Read the model definition and answer for the solid it produces. Units are mm, in the model's axes. Give positions to 0.01 mm unless a question says otherwise; leave off trailing zeros. Loops run counter-clockwise (first coordinate to the right, second up) from the corner with the lowest first, then second, coordinate; pieces in that order, holes last. Notation, with made-up numbers: (30.25, 78) -> (89.25, 78) arc R24 cw to (89.25, 97) -> close; hole circle Ø6 at (-24.5, 0). An arc over 180 degrees is marked (long way). Write each question's results on one line, items separated by ' | '. Start each with the question number.
Item 1: Each of these flat-tipped pins is pushed along its axis until it touches: P1, Ø3, axis at x = -62.76, y = -56.51, coming from the -Z side; P2, Ø0.6, axis at x = 79.5, z = 2, coming from the +Y side; P3, Ø6.5, axis at x = 62.76, y = -56.51, coming from the -Z side; P4, Ø1, axis at x = -24.5, z = 0.5, coming from the +Y side. Where does it stop, or does it pass through?
Item 2: Section A-A on y = 0 is taken. Write down the section's boundary in (x, z) (1 decimal).
Item 3: Find the intervals of material crossed by line 1 (X direction, y = 1.5, z = 0.15); line 2 (Y direction, x = -77, z = 1.4); line 3 (Y direction, x = -57.5, z = 1.1), in increasing order.
Item 4: Section B-B on x = 24.5 is taken. Write down the section's boundary in (y, z) (3 decimals), and give its area (3 significant figures).
Item 5: Section C-C on z = 1.35 is taken. State how many separate pieces and enclosed holes the cut face has, and give its area (3 significant figures).
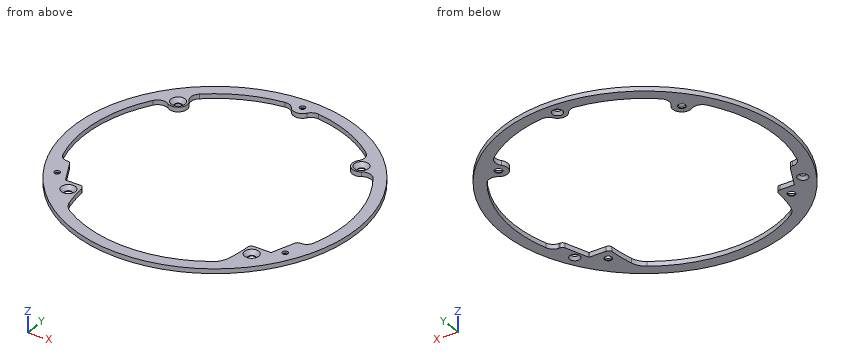
```python
from build123d import *

# Parameters (mm, degrees)
SKETCH1_R                 = 98.1075
SKETCH1_R_2               = 90.17
BOSS_EXTRUDE1_DEPTH       = 3.175
BOSS_EXTRUDE2_START       = -3.175
BOSS_EXTRUDE2_DEPTH       = 3.175
BOSS_EXTRUDE3_START       = -3.175
BOSS_EXTRUDE3_DEPTH       = 3.175
BOSS_EXTRUDE5_DEPTH       = 3.175
MIRROR2_START             = -3.175
MIRROR2_COPY_1_DEPTH      = 3.175
CIRPATTERN1_COUNT         = 3
FILLET1_R                 = 3.175
BOSS_EXTRUDE6_START       = -3.175
BOSS_EXTRUDE6_DEPTH       = 3.175
FILLET2_R                 = 6.35
F_6_CLEARANCE_HOLE1_D     = 3.7973
F_6_CLEARANCE_HOLE1_DEPTH = 6.35
F_6_CLEARANCE_HOLE1_TIP   = 1.140824014
CUT_EXTRUDE1_DEPTH        = 139.781280213
FILLET3_R                 = 2.54


with BuildPart() as part:
    # Sketch1 → Boss-Extrude1 (new body)
    with BuildSketch(Plane.XY):
        Circle(SKETCH1_R)
        Circle(SKETCH1_R_2, mode=Mode.SUBTRACT)
    extrude(amount=BOSS_EXTRUDE1_DEPTH)

    # Sketch2 → Boss-Extrude2 (add)
    with BuildSketch(Plane.XY.offset(3.175).offset(BOSS_EXTRUDE2_START)):
        with BuildLine():
            ThreePointArc((-5.291472464, 86.659612676), (0, 83.82), (5.291472464, 86.659612676))
            ThreePointArc((5.291472464, 86.659612676), (7.940261692, 88.923194985), (11.38468318, 89.448409091))
            ThreePointArc((11.38468318, 89.448409091), (0, 90.17), (-11.38468318, 89.448409091))
            ThreePointArc((-11.38468318, 89.448409091), (-7.940261692, 88.923194985), (-5.291472464, 86.659612676))
        make_face()
    boss_extrude2 = extrude(amount=BOSS_EXTRUDE2_DEPTH)

    # Sketch9 → Boss-Extrude3 (add)
    with BuildSketch(Plane.XY.offset(3.175).offset(BOSS_EXTRUDE3_START)):
        with BuildLine():
            ThreePointArc((66.212341469, -51.332340799), (58.137705987, -52.347425597), (57.972211169, -60.483932635))
            ThreePointArc((57.972211169, -60.483932635), (59.462085873, -65.336411741), (57.068521986, -69.812697257))
            ThreePointArc((57.068521986, -69.812697257), (67.009368913, -60.335506775), (75.395540901, -49.458480691))
            ThreePointArc((75.395540901, -49.458480691), (71.1939725, -52.306831631), (66.212341469, -51.332340799))
        make_face()
    boss_extrude3 = extrude(amount=BOSS_EXTRUDE3_DEPTH)

    # Sketch11 → Boss-Extrude5 (add)
    with BuildSketch(Plane.XY):
        with BuildLine():
            ThreePointArc((-60.552516274, -19.396575562), (-63.5, -44.45), (-60.552516274, -69.503424438))
            ThreePointArc((-60.552516274, -69.503424438), (-57.572960629, -76.08635224), (-52.356101558, -81.086059404))
            ThreePointArc((-52.356101558, -81.086059404), (0, -96.52), (52.356101558, -81.086059404))
            ThreePointArc((52.356101558, -81.086059404), (57.572960629, -76.08635224), (60.552516274, -69.503424438))
            ThreePointArc((60.552516274, -69.503424438), (63.5, -44.45), (60.552516274, -19.396575562))
            ThreePointArc((60.552516274, -19.396575562), (57.572960629, -12.81364776), (52.356101558, -7.813940596))
            ThreePointArc((52.356101558, -7.813940596), (0, 7.62), (-52.356101558, -7.813940596))
            ThreePointArc((-52.356101558, -7.813940596), (-57.572960629, -12.81364776), (-60.552516274, -19.396575562))
        make_face()
        with BuildLine():
            ThreePointArc((48.911621193, -13.148549768), (0, 1.27), (-48.911621193, -13.148549768))
            ThreePointArc((-48.911621193, -13.148549768), (-52.38952724, -16.481687877), (-54.37589767, -20.870306412))
            ThreePointArc((-54.37589767, -20.870306412), (-57.15, -44.45), (-54.37589767, -68.029693588))
            ThreePointArc((-54.37589767, -68.029693588), (-52.38952724, -72.418312123), (-48.911621193, -75.751450232))
            ThreePointArc((-48.911621193, -75.751450232), (0, -90.17), (48.911621193, -75.751450232))
            ThreePointArc((48.911621193, -75.751450232), (52.38952724, -72.418312123), (54.37589767, -68.029693588))
            ThreePointArc((54.37589767, -68.029693588), (57.15, -44.45), (54.37589767, -20.870306412))
            ThreePointArc((54.37589767, -20.870306412), (52.38952724, -16.481687877), (48.911621193, -13.148549768))
        make_face(mode=Mode.SUBTRACT)
    extrude(amount=BOSS_EXTRUDE5_DEPTH)

    # Sketch3 → CSK for #10 Flat Head Machine Screw1 (revolve, cut)
    with BuildSketch(Plane(origin=(62.762296236, -56.51142536, 3.175), x_dir=(0, -1, 0), z_dir=(1, 0, 0))):
        Polygon((0, 0), (0, 3.175), (2.5527, 3.175), (2.5527, 2.688180894), (4.8895, 0), align=None)
    csk_for_10_flat_head_machine_screw1 = revolve(axis=Axis((62.762296236, -56.51142536, 9.525), (0, 0, -1)), mode=Mode.SUBTRACT)

    # Sketch7 → CSK for #6 Flat Head Machine Screw1 (revolve, cut)
    with BuildSketch(Plane(origin=(0, 90.17, 0), x_dir=(0, 1, 0), z_dir=(1, 0, 0))):
        Polygon((0, 0), (0, 3.175), (1.89865, 3.175), (1.89865, 1.891953401), (3.5433, 0), align=None)
    csk_for_6_flat_head_machine_screw1 = revolve(axis=Axis((0, 90.17, -6.35), (0, 0, 1)), mode=Mode.SUBTRACT)

    # Mirror1: Boss-Extrude3, CSK for #10 Flat Head Machine Screw1 across plane
    add(boss_extrude3.mirror(Plane.ZX))
    add(csk_for_10_flat_head_machine_screw1.mirror(Plane.ZX), mode=Mode.SUBTRACT)

    # Mirror2: Boss-Extrude3, CSK for #10 Flat Head Machine Screw1 across plane
    add(boss_extrude3.mirror(Plane(origin=(0, 0, 0), x_dir=(0, 0, 1), z_dir=(1, 0, 0))))
    add(csk_for_10_flat_head_machine_screw1.mirror(Plane(origin=(0, 0, 0), x_dir=(0, 0, 1), z_dir=(1, 0, 0))), mode=Mode.SUBTRACT)

    # Mirror2 copy 1 sketch → Mirror2 copy 1 (add)
    with BuildSketch(Plane(origin=(0, 0, 3.175), x_dir=(-1, 0, 0), z_dir=(0, 0, 1)).offset(MIRROR2_START)):
        with BuildLine():
            ThreePointArc((66.212341469, -51.332340799), (58.137705987, -52.347425597), (57.972211169, -60.483932635))
            ThreePointArc((57.972211169, -60.483932635), (59.462085873, -65.336411741), (57.068521986, -69.812697257))
            ThreePointArc((57.068521986, -69.812697257), (67.009368913, -60.335506775), (75.395540901, -49.458480691))
            ThreePointArc((75.395540901, -49.458480691), (71.1939725, -52.306831631), (66.212341469, -51.332340799))
        make_face()
    extrude(amount=MIRROR2_COPY_1_DEPTH)

    # Mirror2 copy 2 sketch → Mirror2 copy 2 (revolve, cut)
    with BuildSketch(Plane(origin=(-62.762296236, 56.51142536, 3.175), x_dir=(0, 1, 0), z_dir=(-1, 0, 0))):
        Polygon((0, 0), (0, 3.175), (2.5527, 3.175), (2.5527, 2.688180894), (4.8895, 0), align=None)
    revolve(axis=Axis((-62.762296236, 56.51142536, 9.525), (0, 0, -1)), mode=Mode.SUBTRACT)

    # CirPattern1: Boss-Extrude2, CSK for #6 Flat Head Machine Screw1 ×3 about axis
    cirpattern1_axis = Axis((0, 0, 0), (0, 0, 1))
    add([boss_extrude2.rotate(cirpattern1_axis, i * 360 / CIRPATTERN1_COUNT) for i in range(1, CIRPATTERN1_COUNT)])
    add([csk_for_6_flat_head_machine_screw1.rotate(cirpattern1_axis, i * 360 / CIRPATTERN1_COUNT) for i in range(1, CIRPATTERN1_COUNT)], mode=Mode.SUBTRACT)

    # Fillet1
    fillet1_edges = [part.edges().sort_by_distance(p)[0] for p in [
        (-63.34053847, -50.315348785, 1.5875),
        (63.34053847, -50.315348785, 1.5875),
    ]]
    fillet(fillet1_edges, radius=FILLET1_R)

    # Sketch13 → Boss-Extrude6 (add)
    with BuildSketch(Plane.XY.offset(3.175).offset(BOSS_EXTRUDE6_START)):
        with BuildLine():
            Line((-62.750338152, -31.75), (-84.395298447, -31.75))
            ThreePointArc((-84.395298447, -31.75), (-83.790591931, -33.31314461), (-83.156936191, -34.864779698))
            ThreePointArc((-83.156936191, -34.864779698), (-80.979876688, -37.585129154), (-77.695162292, -38.747256761))
            ThreePointArc((-77.695162292, -38.747256761), (-72.590249345, -41.91), (-72.403689828, -47.912355915))
            ThreePointArc((-72.403689828, -47.912355915), (-72.988143244, -49.736636134), (-73.00196491, -51.652202127))
            ThreePointArc((-73.00196491, -51.652202127), (-69.562842084, -52.432853205), (-66.212341469, -51.332340799))
            ThreePointArc((-66.212341469, -51.332340799), (-65.774776399, -51.066180438), (-65.316806621, -50.836902852))
            ThreePointArc((-65.316806621, -50.836902852), (-63.927038857, -49.623372793), (-63.44669601, -47.841974356))
            ThreePointArc((-63.44669601, -47.841974356), (-63.39906785, -39.78298126), (-62.750338152, -31.75))
        make_face()
        with BuildLine():
            Line((84.395298447, -31.75), (62.750338152, -31.75))
            ThreePointArc((62.750338152, -31.75), (63.39906785, -39.78298126), (63.44669601, -47.841974356))
            ThreePointArc((63.44669601, -47.841974356), (63.927038857, -49.623372793), (65.316806621, -50.836902852))
            ThreePointArc((65.316806621, -50.836902852), (65.774776399, -51.066180438), (66.212341469, -51.332340799))
            ThreePointArc((66.212341469, -51.332340799), (69.562842084, -52.432853205), (73.00196491, -51.652202127))
            ThreePointArc((73.00196491, -51.652202127), (72.988143244, -49.736636134), (72.403689828, -47.912355915))
            ThreePointArc((72.403689828, -47.912355915), (72.590249345, -41.91), (77.695162292, -38.747256761))
            ThreePointArc((77.695162292, -38.747256761), (80.979876688, -37.585129154), (83.156936191, -34.864779698))
            ThreePointArc((83.156936191, -34.864779698), (83.790591931, -33.31314461), (84.395298447, -31.75))
        make_face()
    extrude(amount=BOSS_EXTRUDE6_DEPTH)

    # Fillet2
    fillet2_edges = [part.edges().sort_by_distance(p)[0] for p in [
        (-62.750338152, -31.75, 1.5875),
        (-84.395298447, -31.75, 1.5875),
        (84.395298447, -31.75, 1.5875),
        (62.750338152, -31.75, 1.5875),
    ]]
    fillet(fillet2_edges, radius=FILLET2_R)

    # #6 Clearance Hole1
    with Locations(Plane.XY.offset(3.175)):
        with Locations((-66.675, -44.45), (66.675, -44.45)):
            Hole(F_6_CLEARANCE_HOLE1_D / 2, depth=F_6_CLEARANCE_HOLE1_DEPTH)
            with Locations((0, 0, -(F_6_CLEARANCE_HOLE1_DEPTH + F_6_CLEARANCE_HOLE1_TIP / 2))):  # 118° drill point
                Cone(0, F_6_CLEARANCE_HOLE1_D / 2, F_6_CLEARANCE_HOLE1_TIP, mode=Mode.SUBTRACT)

    # Sketch16 → Cut-Extrude1 (cut, through all)
    with BuildSketch(Plane.XY.offset(3.175)):
        Polygon((-79.573670406, -28.758087868), (-69.516837715, -49.335914757), (-54.97311044, -49.335914757), (71.200840815, -49.335914757), (78.661378441, -28.758087868), (74.931109628, 37.993907033), (-79.573670406, 37.993907033), align=None)
    extrude(amount=-CUT_EXTRUDE1_DEPTH, mode=Mode.SUBTRACT)

    # Fillet3
    fillet3_edges = [part.edges().sort_by_distance(p)[0] for p in [
        (77.576653938, -31.75, 1.5875),
        (-78.111457709, -31.75, 1.5875),
        (57.032450882, -49.335914757, 1.5875),
        (-57.032450882, -49.335914757, 1.5875),
    ]]
    fillet(fillet3_edges, radius=FILLET3_R)


solid = part.part
```
Findings:
1) P1: through | P2: y = 57.9 | P3: z = 0 | P4: y = 95.13
2) outline: (-98.1, 0) -> (-90.2, 0) -> (-90.2, 3.2) -> (-98.1, 3.2) -> close; (90.2, 0) -> (98.1, 0) -> (98.1, 3.2) -> (90.2, 3.2) -> close
3) line 1: -98.1 to -90.16, 90.16 to 98.1 | line 2: -60.8 to -47.14, -43.03 to -34.02, 46.92 to 60.8 | line 3: -79.49 to -50.22, 53.19 to 59.83, 69.43 to 79.49
4) outline: (-94.999, 0) -> (-86.778, 0) -> (-86.778, 3.175) -> (-94.999, 3.175) -> close; (86.778, 0) -> (94.999, 0) -> (94.999, 3.175) -> (86.778, 3.175) -> close | area: 52.2 mm2
5) separate pieces: 1 | enclosed holes: 8 | area: 5,590 mm2
